```python
from build123d import *

# Parameters (mm, degrees)
F0_W     = 100
F0_H     = 100
F1_DEPTH = 200
F2_R     = 33.3715216042
F3_DEPTH = 273
F4_R     = 5


with BuildPart() as f1:
    # F0 (on Front) → F1 (new body)
    with BuildSketch(Plane.XZ):
        Rectangle(F0_W, F0_H)
    extrude(amount=F1_DEPTH)

    # F2 (on face) → F3 (cut)
    with BuildSketch(Plane.XZ.offset(200)):
        Circle(F2_R)
    extrude(amount=-F3_DEPTH, mode=Mode.SUBTRACT)

    # F4
    f4_edges = [f1.edges().sort_by_distance(p)[0] for p in [
        (50, -100, 50),
        (-50, -100, 50),
        (0, 0, 50),
        (0, -200, 50),
        (-50, -100, -50),
        (-50, 0, 0),
        (-50, -200, 0),
        (50, 0, 0),
        (0, 0, -50),
        (-33.371522, 0, 0),
        (50, -100, -50),
        (50, -200, 0),
        (0, -200, -50),
        (-33.371522, -200, 0),
    ]]
    fillet(f4_edges, radius=F4_R)


solid = f1.part
```
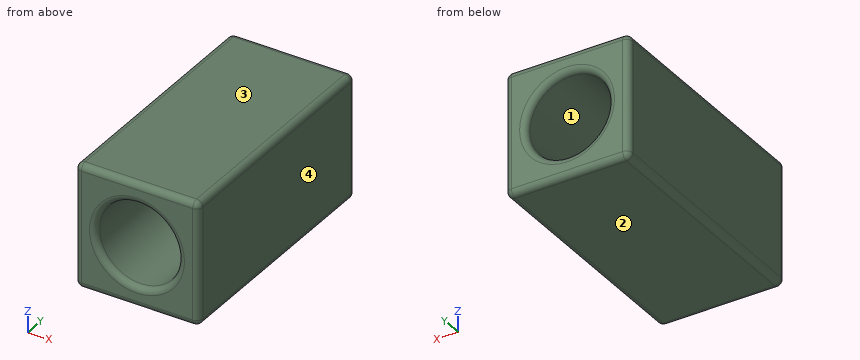
Geometry check sheet. Reference: the model listing, model coordinates, mm. Face numbers are marked on the shaded views. Round coordinates to 2 decimals unless told otherwise and drop trailing zeros. Loops run counter-clockwise (first coordinate to the right, second up) from the corner with the lowest first, then second, coordinate; pieces in that order, holes last. Notation, with made-up numbers: (42, 26) - (90, 26) arc R36 cw to (90, 65) - close; hole circle Ø1 at (59.25, -22.5). An arc over 180 degrees is marked (long way). Use a Markdown table: item, result.
Q1. Material ranges on line 1 (Z direction, x = 0, y = -76); line 2 (X direction, y = -140.5, z = 7); line 3 (Z direction, x = 24, y = -13), recorded low to high.
Solutions:
| item | result |
|---|---|
| line 1 | z = -50 to -33.37, 33.37 to 50 |
| line 2 | x = -50 to -32.63, 32.63 to 50 |
| line 3 | z = -50 to -23.19, 23.19 to 50 |
Q2. Cross-section at C-C on y = -111. Record the cut outline in (x, z).
Solutions:
| item | result |
|---|---|
| outline | (-50, -45) arc R5 ccw to (-45, -50) - (45, -50) arc R5 ccw to (50, -45) - (50, 45) arc R5 ccw to (45, 50) - (-45, 50) arc R5 ccw to (-50, 45) - close; hole circle Ø66.74 at (0, 0) |
Q3. Cross-section at A-A on z = 0. Record the cut outline in (x, y), plus the area to 3 significant figures.
Solutions:
| item | result |
|---|---|
| outline | (-50, -195) arc R5 ccw to (-45, -200) - (-38.37, -200) arc R5 ccw to (-33.37, -195) - (-33.37, -5) arc R5 ccw to (-38.37, 0) - (-45, 0) arc R5 ccw to (-50, -5) - close; (33.37, -195) arc R5 ccw to (38.37, -200) - (45, -200) arc R5 ccw to (50, -195) - (50, -5) arc R5 ccw to (45, 0) - (38.37, 0) arc R5 ccw to (33.37, -5) - close |
| area | 6,610 mm2 |
Q4. Cross-section at B-B on x = 0. Record the cut outline in (y, z), plus the area to 3 significant figures.
Solutions:
| item | result |
|---|---|
| outline | (-200, -45) arc R5 ccw to (-195, -50) - (-5, -50) arc R5 ccw to (0, -45) - (0, -38.37) arc R5 ccw to (-5, -33.37) - (-195, -33.37) arc R5 ccw to (-200, -38.37) - close; (-200, 38.37) arc R5 ccw to (-195, 33.37) - (-5, 33.37) arc R5 ccw to (0, 38.37) - (0, 45) arc R5 ccw to (-5, 50) - (-195, 50) arc R5 ccw to (-200, 45) - close |
| area | 6,610 mm2 |
Q5. Draft check along Z on the marked faces 1, 2, 3 and 4. Enter one of: released by +Z, released by -Z, zero draft, split by the parting line, or undercut.
Solutions:
| item | result |
|---|---|
| face 1 | undercut |
| face 2 | released by -Z |
| face 3 | released by +Z |
| face 4 | zero draft |
